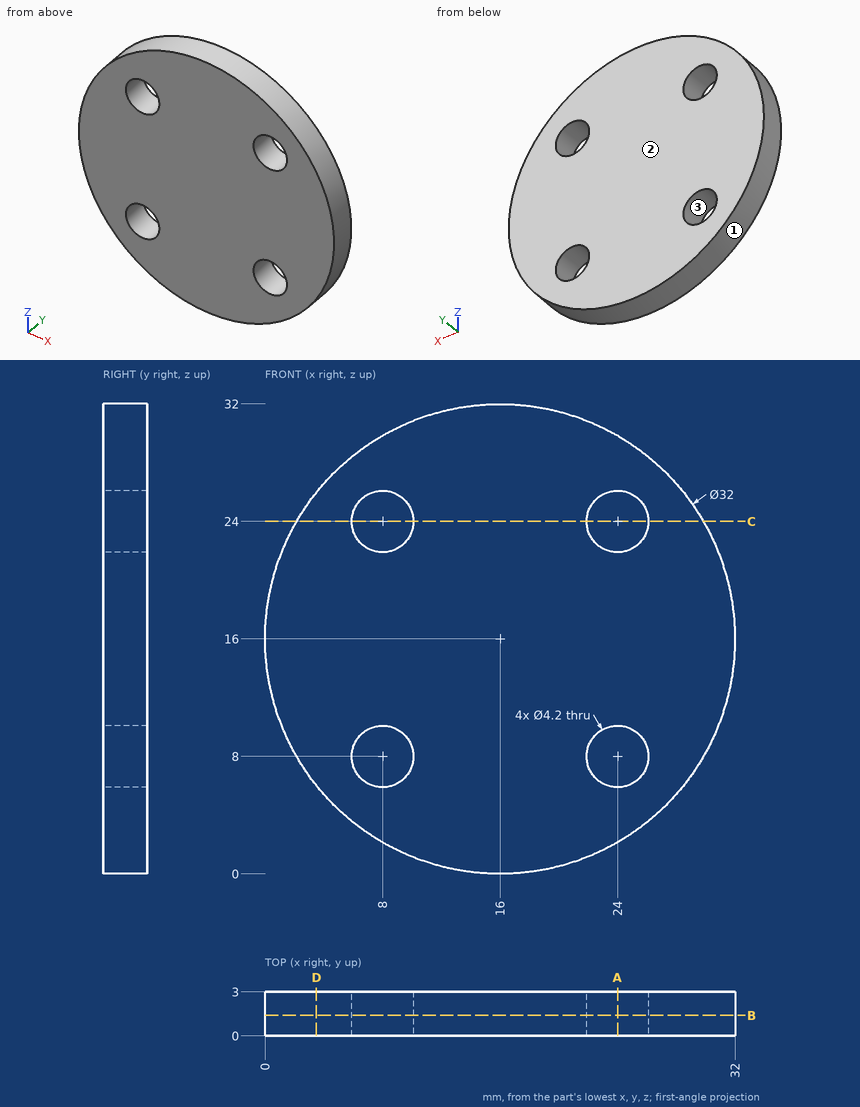
Geometry check sheet. Reference: drawing and pictorial views, mm from the part's lowest x, y, z. Coordinates: 2 decimals unless noted, no trailing zeros. Write each loop counter-clockwise with the first axis right and the second up, starting at its lowest first coordinate (ties: lowest second). Pieces come first, ordered by that corner, then holes. Notation, with made-up numbers: M 3.5,-36.5 L 10.5,-36.5 A24 ccw 10.5,-6.5 Z; hole C 71,-28.5 d5. An arc over 180 degrees is marked long. Write item = value, one per line. Start each with the question number.
1. Sectioned sample at C-C (z = 24). Record the cut outline in (x, y).
2. Go/stop test with flat-tipped pins: pin 1 (1.5 mm diameter, centred on x = 23, y = 1.5, fed in from -Z); pin 2 (2.5 mm diameter, centred on x = 8, z = 8, fed in from +Y); pin 3 (1 mm diameter, centred on y = 0.5, z = 13.5, fed in from +X). Record where each tip stops, or that it passes through.
3. Thickness scan on probe 1 along X at (y, z) = (2.8, 9); probe 2 along Z at (x, y) = (7.5, 2.5). Record the ranges inside material, lowest first.
4. Sectioned sample at D-D (x = 3.5). Record the cut outline in (y, z).
5. Mould release check, pull along X, two halves, no side actions. Record for the marked faces 1, 2 and 3: pulls with the +X half, pulls with the -X half, needs draft (parallel to the pull), parting line crosses it, or undercut.
6. Sectioned sample at B-B (y = 1.4). Record the cut outline in (x, z), then the cut area to 3 significant figures.
7. Sectioned sample at A-A (x = 24). Record the cut outline in (y, z), then the cut area to 3 significant figures.
The answers:
q1.outline = M 2.14,0 L 5.9,0 L 5.9,3 L 2.14,3 Z; M 10.1,0 L 21.9,0 L 21.9,3 L 10.1,3 Z; M 26.1,0 L 29.86,0 L 29.86,3 L 26.1,3 Z
q2.pin_1 = 1.27
q2.pin_2 = through
q2.pin_3 = 31.87
q3.probe_1 = 1.61 to 6.15, 9.85 to 22.15, 25.85 to 30.39
q3.probe_2 = 2.44 to 5.96, 10.04 to 21.96, 26.04 to 29.56
q4.outline = M 0,6.01 L 3,6.01 L 3,25.99 L 0,25.99 Z
q5.face_1 = parting line crosses it
q5.face_2 = needs draft
q5.face_3 = undercut
q6.outline = C 16,16 d32; hole C 8,8 d4.2; hole C 8,24 d4.2; hole C 24,8 d4.2; hole C 24,24 d4.2
q6.area = 749 mm²
q7.outline = M 0,2.14 L 3,2.14 L 3,5.9 L 0,5.9 Z; M 0,10.1 L 3,10.1 L 3,21.9 L 0,21.9 Z; M 0,26.1 L 3,26.1 L 3,29.86 L 0,29.86 Z
q7.area = 57.9 mm²
